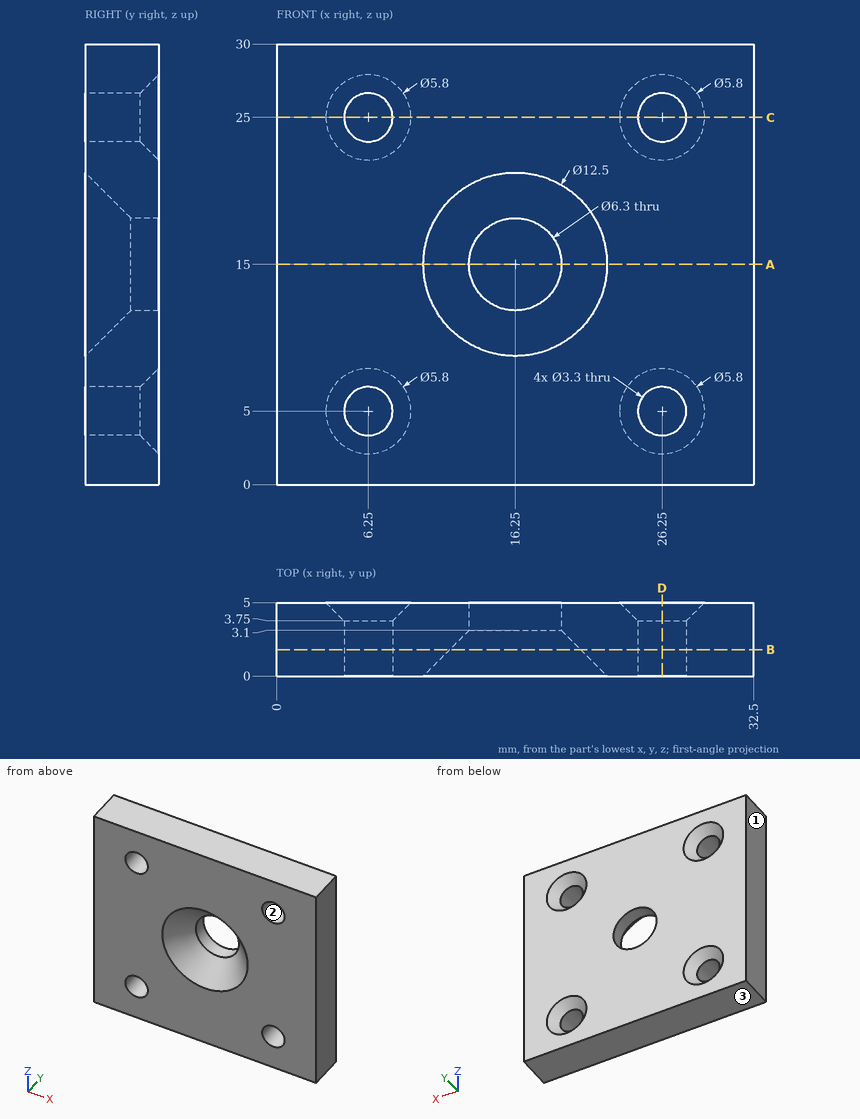
Can you work these out from the drawing? Everything is in mm from the part's minimum corner. Round coordinates to 2 decimals unless told otherwise and drop trailing zeros. Write each loop counter-clockwise with the first axis right and the second up, starting at its lowest first coordinate (ties: lowest second). Pieces come first, ordered by that corner, then holes. Notation, with made-up numbers: M 61.5,1 L 77.5,1 A18 ccw 77.5,10 Z; hole C 84.5,70 d10. An arc over 180 degrees is marked long. Use a Markdown table: item, result.
Item 1: We'd pull the mould along X, two halves only. Please class the marked faces 1, 2 and 3: released by +X, released by -X, zero draft, split by the parting line, or undercut.
Found:
| item | result |
|---|---|
| face 1 | released by -X |
| face 2 | undercut |
| face 3 | zero draft |
Item 2: If I drill on line 1 along X through (y, z) = (1.2, 5); line 2 along Z through (x, y) = (26.25, 1.65); line 3 along X through (y, z) = (4.6, 15), over which ranges is the centre line in solid material (lowest first)? Write a range as [from, to].
Found:
| item | result |
|---|---|
| line 1 | x = [0, 4.6], [7.9, 24.6], [27.9, 32.5] |
| line 2 | z = [0, 3.35], [6.65, 23.35], [26.65, 30] |
| line 3 | x = [0, 13.1], [19.4, 32.5] |
Item 3: I want a section at C-C (z = 25). List the corners of the cut face in (x, y) for me.
Found:
| item | result |
|---|---|
| outline | M 0,0 L 4.6,0 L 4.6,3.75 L 3.35,5 L 0,5 Z; M 7.9,0 L 24.6,0 L 24.6,3.75 L 23.35,5 L 9.15,5 L 7.9,3.75 Z; M 27.9,0 L 32.5,0 L 32.5,5 L 29.15,5 L 27.9,3.75 Z |
Item 4: I want a section at A-A (z = 15). List the corners of the cut face in (x, y) for me.
Found:
| item | result |
|---|---|
| outline | M 0,0 L 10,0 L 13.1,3.1 L 13.1,5 L 0,5 Z; M 19.4,3.1 L 22.5,0 L 32.5,0 L 32.5,5 L 19.4,5 Z |
Item 5: For pin 1 Ø4.5 at (x, z) = (26.25, 5) entering from +Y; pin 2 Ø7 at (x, z) = (16.25, 15) entering from -Y, each with a flat end and sliding along its axis, tell me the tip position at first contact or that it passes through.
Found:
| item | result |
|---|---|
| pin 1 | stops at y = 4.35 |
| pin 2 | stops at y = 2.75 |
Item 6: I want a section at D-D (x = 26.25). List the corners of the cut face in (y, z) for me.
Found:
| item | result |
|---|---|
| outline | M 0,0 L 5,0 L 5,2.1 L 3.75,3.35 L 0,3.35 Z; M 0,6.65 L 3.75,6.65 L 5,7.9 L 5,22.1 L 3.75,23.35 L 0,23.35 Z; M 0,26.65 L 3.75,26.65 L 5,27.9 L 5,30 L 0,30 Z |
Item 7: I want a section at B-B (y = 1.8). List the corners of the cut face in (x, z) for me, and give its area (3 significant figures).
Found:
| item | result |
|---|---|
| outline | M 0,0 L 32.5,0 L 32.5,30 L 0,30 Z; hole C 6.25,5 d3.3; hole C 6.25,25 d3.3; hole C 16.25,15 d8.9; hole C 26.25,5 d3.3; hole C 26.25,25 d3.3 |
| area | 879 mm2 |
